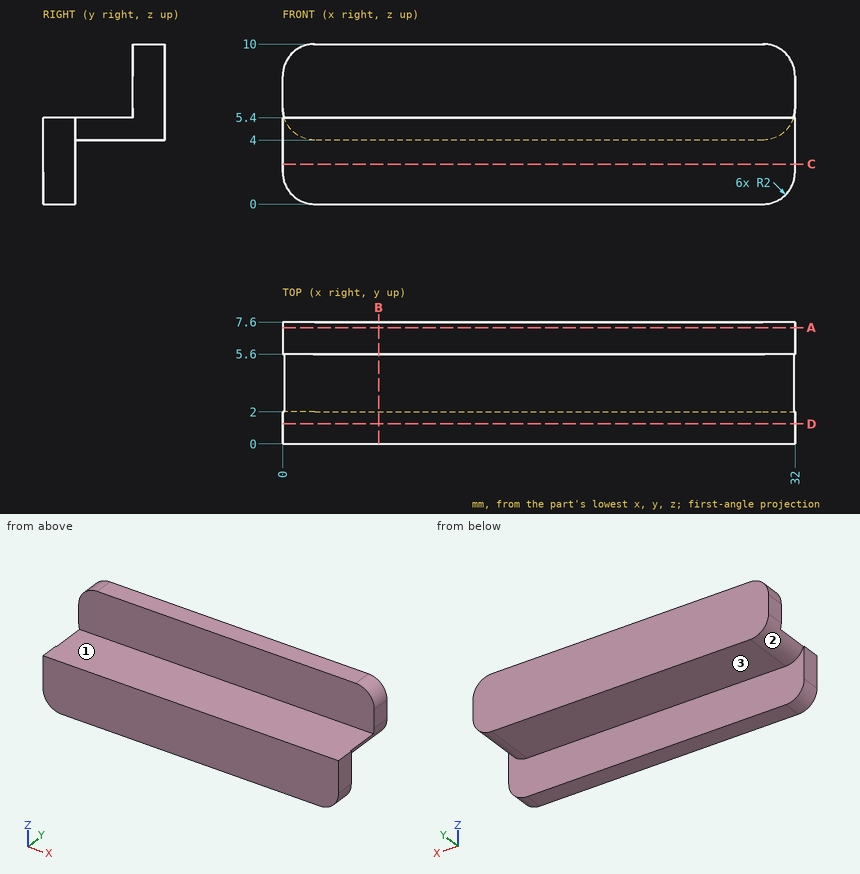
Here's the drawing with two shaded views (mm, measured from the low corner). I have some questions. A direction names the side the tool comes from. Round coordinates to 2 decimals unless told otherwise and drop trailing zeros. Loops run counter-clockwise (first coordinate to the right, second up) from the corner with the lowest first, then second, coordinate; pieces in that order, holes last. Notation, with made-up numbers: M 63,-24 L 122,-24 A18 ccw 122,-19 Z; hole C 0.5,71 d10. An arc over 180 degrees is marked long. Answer as a JSON object with one key per item and string values. Group by question number.
Q1. Imagine slicing it at C-C, the plane z = 2.5. Please give me the cut outline in (x, y), then the cut area to 3 significant figures.
Q2. Imagine slicing it at D-D, the plane y = 1.25. Please give me the cut outline in (x, z), then the cut area to 3 significant figures.
Q3. Imagine slicing it at B-B, the plane x = 6. Please give me the cut outline in (y, z).
Q4. Will these pins go through, and if not, where does the flat tip stop? pin 1 (1.5 mm diameter, centred on x = 10, y = 2, fed in from +Z); pin 2 (2.5 mm diameter, centred on x = 13.5, z = 7.5, fed in from -Y); pin 3 (1.6 mm diameter, centred on x = 21, z = 2, fed in from +Y).
Q5. Please list where these lines run through material, in increasing order: L1, parallel to Z at x = 13.5, y = 3; L2, parallel to Y at x = 27.5, z = 9.75; L3, parallel to Z at x = 7.5, y = 1.5.
Q6. On a 3-axis mill with a long thin cutter (end or side, diameter ignored), from which of +Z, -Z, +X, -X, +Y, -Y can I reach the whole of each face in a straight line? I mean the marked faces 1, 2 and 3. Say none if no direction works.
Q7. Imagine slicing it at A-A, the plane y = 7.25. Please give me the cut outline in (x, z).
Findings:
{
 "1": {"outline": "M 0,0 L 32,0 L 32,2 L 0,2 Z", "area": "64.0 mm2"},
 "2": {"outline": "M 0,2 A2 ccw 2,0 L 30,0 A2 ccw 32,2 L 32,5.4 L 0,5.4 Z", "area": "171 mm2"},
 "3": {"outline": "M 0,0 L 2,0 L 2,4 L 7.6,4 L 7.6,10 L 5.6,10 L 5.6,5.4 L 0,5.4 Z"},
 "4": {"pin 1": "stops at z = 5.4", "pin 2": "stops at y = 5.6", "pin 3": "stops at y = 2"},
 "5": {"L1": "z = 4 to 5.4", "L2": "y = 5.6 to 7.6", "L3": "z = 0 to 5.4"},
 "6": {"face 1": "+Z, +X, -X, -Y", "face 2": "-Z, -X, +Y", "face 3": "-Z, +X, -X, +Y"},
 "7": {"outline": "M 0,6 A2 ccw 2,4 L 30,4 A2 ccw 32,6 L 32,8 A2 ccw 30,10 L 2,10 A2 ccw 0,8 Z"}
}
